```python
from build123d import *

# Parameters (mm, degrees)
F0_R     = 6.717517972
F0_R_2   = 6.020799142
F0_W     = 93.3380946517
F0_H     = 25.1572784036
F1_DEPTH = 25.4
F2_R     = 6.1623070593
F2_R_2   = 6.4550817185
F3_DEPTH = 19.05
F4_R     = 5.08


with BuildPart() as f1:
    # F0 (on Right) → F1 (new body)
    with BuildSketch(Plane.YZ):
        Polygon((-29.2035490274, 0), (-63.4982287884, 0), (-63.4982287884, -35.7638783753), (64.1345456243, -72.88698107), (64.1345456243, -25.1572784036), (-29.2035490274, -25.1572784036), align=None)
        with Locations((46.4568771422, -50.9666763246)):
            Circle(F0_R, mode=Mode.SUBTRACT)
        with Locations((-47.2347699106, -16.3184423)):
            Circle(F0_R_2, mode=Mode.SUBTRACT)
        with Locations((17.4654982984, -12.5786392018)):
            Rectangle(F0_W, F0_H)
    extrude(amount=F1_DEPTH)

    # F2 (on Top) → F3 (join)
    with BuildSketch(Plane.XY):
        with BuildLine():
            Line((-49.083184828, 53.9312161083), (-64.3051586518, -21.9885608041))
            ThreePointArc((-64.3051586518, -21.9885608041), (-61.737725203, -32.4590575274), (-52.0475044965, -37.1837415174))
            Line((-52.0475044965, -37.1837415174), (25.4, -37.1837415174))
            Line((25.4, -37.1837415174), (25.4, 64.1345456243))
            Line((25.4, 64.1345456243), (-36.6310108614, 64.1345456243))
            ThreePointArc((-36.6310108614, 64.1345456243), (-44.6803053911, 61.2579288283), (-49.083184828, 53.9312161083))
        make_face()
        with Locations((-51.8529846852, -24.4852312881)):
            Circle(F2_R, mode=Mode.SUBTRACT)
        with Locations((-36.6310108614, 51.4345456243)):
            Circle(F2_R_2, mode=Mode.SUBTRACT)
    extrude(amount=-F3_DEPTH)

    # F4
    f4_edges = [f1.edges().sort_by_distance(p)[0] for p in [
        (12.7, 64.134546, -72.886981),
        (12.7, -63.498229, -35.763878),
        (12.7, -63.498229, 0),
        (0, 13.475402, -19.05),
    ]]
    fillet(f4_edges, radius=F4_R)


solid = f1.part
```
For this review, take the finished solid that the model builds, in its own axes (mm). A direction names the side the tool comes from. Coordinates: 2 decimals unless noted, no trailing zeros. Write each loop counter-clockwise with the first axis right and the second up, starting at its lowest first coordinate (ties: lowest second). Pieces come first, ordered by that corner, then holes.
(1) Add section D-D on x = -16.5. Give the boundary of the cut face in (y, z), then the cut area to 3 significant figures.
(2) The part is to be moulded in two halves that separate along Y. For faces 4 (the face through (12.88, -62.51, -34.96)), 5 (the face through (2, 64.135, -25)), 6 (the face through (12.522, 41.506, -46.427)), say which applies: +Y half, -Y half, draft (parallel to the pull), parting line (faces both ways), or undercut.
(3) Add section C-C on z = -13. Give the boundary of the cut face in (x, y).
(4) Add section B-B on y = 56. Give the boundary of the cut face in (x, z), then the cut area to 3 significant figures.
(5) For pin 1 Ø12 at (y, z) = (20, -26.5) entering from -X; pin 2 Ø10 at (x, z) = (-15.5, -20.5) entering from -Y; pin 3 Ø17 at (x, y) = (-36.63, 51.43) entering from -Z, all flat-tipped, find the tip position at first contact; note any pin that passes through.
(6) Wall thickness on probe 1 along Z at (x, y) = (-12, 28.5); probe 2 along X at (y, z) = (25, -38.5); probe 3 along Y at (x, z) = (-32, -13.5): over which ranges is each line inside the solid? List them lowest first.
(7) Tool access review of faces 1 (the face through (-29, 14, -19.05)), 2 (the face through (0, -1, -35)), 3 (the face through (-26, -37.184, -9)): name each direction out of +Z, -Z, +X, -X, +Y, -Y from which nothing blocks a thin tool from reaching the whole face with its end or side.
(8) Add section A-A on z = -53. Give the boundary of the cut face in (x, y), then the cut area to 3 significant figures.
Answer sheet:
1. outline: (-37.18, -19.05) - (64.13, -19.05) - (64.13, 0) - (-37.18, 0) - close
1. area: 1,930 mm2
2. face 4: -Y half
2. face 5: +Y half
2. face 6: undercut
3. outline: (-64.31, -21.99) arc R12.7 ccw to (-52.05, -37.18) - (0, -37.18) - (0, -42.21) - (25.4, -42.21) - (25.4, 64.13) - (-36.63, 64.13) arc R12.7 ccw to (-49.08, 53.93) - close; (0, -63.5) - (25.4, -63.5) - (25.4, -52.26) - (0, -52.26) - close; hole circle Ø12.32 at (-51.85, -24.49); hole circle Ø12.91 at (-36.63, 51.43)
4. outline: (-48.48, -19.05) - (-41.19, -19.05) - (-41.19, 0) - (-48.48, 0) - close; (-32.07, -19.05) - (-5.08, -19.05) arc R5.08 cw to (0, -24.13) - (0, -70.52) - (25.4, -70.52) - (25.4, 0) - (-32.07, 0) - close
4. area: 2,550 mm2
5. pin 1: stops at x = -1.53
5. pin 2: stops at y = -37.18
5. pin 3: stops at z = -19.05
6. probe 1: z = -19.05 to 0
6. probe 2: x = 0 to 25.4
6. probe 3: y = -37.18 to 46.94, 55.93 to 64.13
7. face 1: -Z, -X, +Y, -Y
7. face 2: -Z, -X, -Y
7. face 3: +Z, -Z, -X, -Y
8. outline: (0, -4.24) - (25.4, -4.24) - (25.4, 40.05) - (0, 40.05) - close; (0, 52.86) - (25.4, 52.86) - (25.4, 64.13) - (0, 64.13) - close
8. area: 1,410 mm2
